from build123d import *

# Parameters (mm, degrees)
ESTRUSIONE_ESTRUSIONE2_DEPTH      = 150
ESTRUSIONE_ESTRUSIONE2_DEPTH_BACK = 150
ESTRUSIONE_ESTRUSIONE3_DEPTH      = 3.3
ESTRUSIONE_ESTRUSIONE3_DEPTH_BACK = 303.3
SCHIZZO3_W                        = 6.5
SCHIZZO3_H                        = 6.5
SCHIZZO11_W                       = 60
SCHIZZO11_H                       = 4
ESTRUSIONE_ESTRUSIONE10_DEPTH     = 2.5
ESTRUSIONE_ESTRUSIONE11_DEPTH     = 2.5
SCHIZZO11_8_W                     = 43
SCHIZZO11_8_H                     = 1.75
ESTRUSIONE_ESTRUSIONE12_DEPTH     = 4.5
SCHIZZO13_W                       = 213
SCHIZZO13_H                       = 5
ESTRUSIONE_ESTRUSIONE13_DEPTH     = 300
SCHIZZO15_W                       = 7
SCHIZZO15_H                       = 5
ESTRUSIONE_ESTRUSIONE14_DEPTH     = 4
SCHIZZO16_W                       = 213
SCHIZZO16_H                       = 5
ESTRUSIONE_ESTRUSIONE15_DEPTH     = 300
RIPETIZIONE_A_L2_COUNT            = 2
RIPETIZIONE_A_L2_PITCH            = 304
SPECCHIA2_COPY_1_SKETCH_W         = 7
SPECCHIA2_COPY_1_SKETCH_H         = 5
SPECCHIA2_COPY_1_DEPTH            = 4
SPECCHIA2_COPY_2_SKETCH_W         = 213
SPECCHIA2_COPY_2_SKETCH_H         = 5
SPECCHIA2_COPY_2_DEPTH            = 300
SCHIZZO17_W                       = 83.15
SCHIZZO17_H                       = 226.3
TAGLIO_ESTRUSIONE1_DEPTH          = 404
SCHIZZO18_W                       = 226.3
SCHIZZO18_H                       = 7
SCHIZZO18_H_2                     = 282
TAGLIO_ESTRUSIONE2_DEPTH          = 404
SCHIZZO23_W                       = 221.3
SCHIZZO23_H                       = 4
SCHIZZO23_H_2                     = 1.75
TAGLIO_ESTRUSIONE7_DEPTH          = 404
SCHIZZO24_W                       = 20
SCHIZZO24_H                       = 221.3
TAGLIO_ESTRUSIONE8_DEPTH          = 404


with BuildPart() as part:
    # Schizzo2 → Estrusione-Estrusione2 (new, two sides: drawn at the far end of the back side and taken through both)
    with BuildSketch(Plane(origin=(0, 0, 0), x_dir=(1, 0, 0), z_dir=(0, 1, 0)).offset(-ESTRUSIONE_ESTRUSIONE2_DEPTH_BACK)):
        Polygon((-113.15, 106.65), (-113.15, -106.65), (-106.65, -106.65), (-106.65, -113.15), (106.65, -113.15), (106.65, -106.65), (113.15, -106.65), (113.15, 106.65), (106.65, 106.65), (106.65, 113.15), (-106.65, 113.15), (-106.65, 106.65), align=None)
    extrude(amount=ESTRUSIONE_ESTRUSIONE2_DEPTH + ESTRUSIONE_ESTRUSIONE2_DEPTH_BACK)

    # Schizzo3 → Estrusione-Estrusione3 (add, two sides: drawn at the far end of the back side and taken through both)
    with BuildSketch(Plane.XZ.offset(150).offset(-ESTRUSIONE_ESTRUSIONE3_DEPTH_BACK)):
        with Locations((-109.9, 109.9)):
            Rectangle(SCHIZZO3_W, SCHIZZO3_H)
        with Locations((109.9, 109.9)):
            Rectangle(SCHIZZO3_W, SCHIZZO3_H)
        with Locations((109.9, -109.9)):
            Rectangle(SCHIZZO3_W, SCHIZZO3_H)
        with Locations((-109.9, -109.9)):
            Rectangle(SCHIZZO3_W, SCHIZZO3_H)
    extrude(amount=ESTRUSIONE_ESTRUSIONE3_DEPTH + ESTRUSIONE_ESTRUSIONE3_DEPTH_BACK)

    # Schizzo11 → Estrusione-Estrusione10 (add)
    with BuildSketch(Plane(origin=(0, 0, -113.15), x_dir=(-1, 0, 0), z_dir=(0, 0, -1))):
        with Locations((0, 141)):
            Rectangle(SCHIZZO11_W, SCHIZZO11_H)
    estrusione_estrusione10 = extrude(amount=ESTRUSIONE_ESTRUSIONE10_DEPTH)

    # Schizzo11_5 → Estrusione-Estrusione11 (add)
    with BuildSketch(Plane(origin=(0, 0, -113.15), x_dir=(-1, 0, 0), z_dir=(0, 0, -1))):
        Polygon((30, 139), (-30, 139), (-45, 139), (-45, 135.5), (-43, 135.5), (-43, 133.75), (0, 133.75), (43, 133.75), (43, 135.5), (45, 135.5), (45, 139), align=None)
    estrusione_estrusione11 = extrude(amount=ESTRUSIONE_ESTRUSIONE11_DEPTH)

    # Schizzo11_8 → Estrusione-Estrusione12 (add)
    with BuildSketch(Plane(origin=(0, 0, -113.15), x_dir=(-1, 0, 0), z_dir=(0, 0, -1))):
        with Locations((21.5, 132.875)):
            Rectangle(SCHIZZO11_8_W, SCHIZZO11_8_H)
        with Locations((-21.5, 132.875)):
            Rectangle(SCHIZZO11_8_W, SCHIZZO11_8_H)
        Polygon((-43, 135.5), (-45, 135.5), (-45, 132), (-43, 132), (-43, 133.75), align=None)
        Polygon((45, 132), (45, 135.5), (43, 135.5), (43, 133.75), (43, 132), align=None)
    estrusione_estrusione12 = extrude(amount=ESTRUSIONE_ESTRUSIONE12_DEPTH)

    # Schizzo13 → Estrusione-Estrusione13 (add)
    with BuildSketch(Plane(origin=(0, 0, -115.65), x_dir=(-1, 0, 0), z_dir=(0, 0, -1))):
        with Locations((-0.15, 136.25)):
            Rectangle(SCHIZZO13_W, SCHIZZO13_H)
    estrusione_estrusione13 = extrude(amount=ESTRUSIONE_ESTRUSIONE13_DEPTH)

    # Schizzo15 → Estrusione-Estrusione14 (add)
    with BuildSketch(Plane(origin=(0, 0, -415.65), x_dir=(-1, 0, 0), z_dir=(0, 0, -1))):
        with Locations((-98.15, 136.25)):
            Rectangle(SCHIZZO15_W, SCHIZZO15_H)
        with Locations((98.15, 136.25)):
            Rectangle(SCHIZZO15_W, SCHIZZO15_H)
    estrusione_estrusione14 = extrude(amount=ESTRUSIONE_ESTRUSIONE14_DEPTH)

    # Schizzo16 → Estrusione-Estrusione15 (add)
    with BuildSketch(Plane(origin=(0, 0, -419.65), x_dir=(-1, 0, 0), z_dir=(0, 0, -1))):
        with Locations((-0.15, 136.25)):
            Rectangle(SCHIZZO16_W, SCHIZZO16_H)
    estrusione_estrusione15 = extrude(amount=ESTRUSIONE_ESTRUSIONE15_DEPTH)

    # Ripetizione a L2: Estrusione-Estrusione14, Estrusione-Estrusione15 ×2
    with Locations(*[(0, 0, -i * RIPETIZIONE_A_L2_PITCH) for i in range(1, RIPETIZIONE_A_L2_COUNT)]):
        add(estrusione_estrusione14)
        add(estrusione_estrusione15)

    # Specchia2: Estrusione-Estrusione10, Estrusione-Estrusione11, Estrusione-Estrusione12, Estrusione-Estrusione13, Estrusione-Estrusione14, Estrusione-Estrusione15 across plane
    add(estrusione_estrusione10.mirror(Plane.XY))
    add(estrusione_estrusione11.mirror(Plane.XY))
    add(estrusione_estrusione12.mirror(Plane.XY))
    add(estrusione_estrusione13.mirror(Plane.XY))
    add(estrusione_estrusione14.mirror(Plane.XY))
    add(estrusione_estrusione15.mirror(Plane.XY))

    # Specchia2 copy 1 sketch → Specchia2 copy 1 (add)
    with BuildSketch(Plane(origin=(0, 0, 719.65), x_dir=(-1, 0, 0), z_dir=(0, 0, 1))):
        with Locations((-98.15, -136.25)):
            Rectangle(SPECCHIA2_COPY_1_SKETCH_W, SPECCHIA2_COPY_1_SKETCH_H)
        with Locations((98.15, -136.25)):
            Rectangle(SPECCHIA2_COPY_1_SKETCH_W, SPECCHIA2_COPY_1_SKETCH_H)
    extrude(amount=SPECCHIA2_COPY_1_DEPTH)

    # Specchia2 copy 2 sketch → Specchia2 copy 2 (add)
    with BuildSketch(Plane(origin=(0, 0, 723.65), x_dir=(-1, 0, 0), z_dir=(0, 0, 1))):
        with Locations((-0.15, -136.25)):
            Rectangle(SPECCHIA2_COPY_2_SKETCH_W, SPECCHIA2_COPY_2_SKETCH_H)
    extrude(amount=SPECCHIA2_COPY_2_DEPTH)

    # Schizzo17 → Taglio-Estrusione1 (cut)
    with BuildSketch(Plane(origin=(0, 150, 0), x_dir=(1, 0, 0), z_dir=(0, 1, 0))):
        with Locations((-71.575, 0)):
            Rectangle(SCHIZZO17_W, SCHIZZO17_H)
        with Locations((71.575, 0)):
            Rectangle(SCHIZZO17_W, SCHIZZO17_H)
    extrude(amount=-TAGLIO_ESTRUSIONE1_DEPTH, mode=Mode.SUBTRACT)


with BuildPart() as taglio_estrusione1_piece_1:
    # of the separate pieces the step leaves, piece 1, a body of its own (taglio_estrusione1_pieces)
    add(part.part.solids().sort_by_distance((106.65, 138.75, 723.65))[0])

    # Schizzo18 → Taglio-Estrusione2 (cut)
    with BuildSketch(Plane(origin=(30, 0, 0), x_dir=(0, 0, -1), z_dir=(1, 0, 0))):
        with Locations((0, 146.5)):
            Rectangle(SCHIZZO18_W, SCHIZZO18_H)
        with Locations((0, -9)):
            Rectangle(SCHIZZO18_W, SCHIZZO18_H_2)
    extrude(amount=-TAGLIO_ESTRUSIONE2_DEPTH, mode=Mode.SUBTRACT)

    # Schizzo23 → Taglio-Estrusione7 (cut)
    with BuildSketch(Plane(origin=(30, 0, 0), x_dir=(0, 0, -1), z_dir=(1, 0, 0))):
        with Locations((0, 141)):
            Rectangle(SCHIZZO23_W, SCHIZZO23_H)
        with Locations((0, 132.875)):
            Rectangle(SCHIZZO23_W, SCHIZZO23_H_2)
    extrude(amount=-TAGLIO_ESTRUSIONE7_DEPTH, mode=Mode.SUBTRACT)

    # Schizzo24 → Taglio-Estrusione8 (cut)
    with BuildSketch(Plane(origin=(0, 139, 0), x_dir=(1, 0, 0), z_dir=(0, 1, 0))):
        with Locations((-20, 0)):
            Rectangle(SCHIZZO24_W, SCHIZZO24_H)
        with Locations((20, 0)):
            Rectangle(SCHIZZO24_W, SCHIZZO24_H)
    extrude(amount=-TAGLIO_ESTRUSIONE8_DEPTH, mode=Mode.SUBTRACT)


with BuildPart() as taglio_estrusione1_piece_2:
    # of the separate pieces the step leaves, piece 2, a body of its own (taglio_estrusione1_pieces)
    add(part.part.solids().sort_by_distance((-106.65, 150, 113.15))[0])


with BuildPart() as taglio_estrusione1_piece_3:
    # of the separate pieces the step leaves, piece 3, a body of its own (taglio_estrusione1_pieces)
    add(part.part.solids().sort_by_distance((-106.65, 150, -106.65))[0])


with BuildPart() as taglio_estrusione1_piece_4:
    # of the separate pieces the step leaves, piece 4, a body of its own (taglio_estrusione1_pieces)
    add(part.part.solids().sort_by_distance((113.15, 150, -106.65))[0])


with BuildPart() as taglio_estrusione1_piece_5:
    # of the separate pieces the step leaves, piece 5, a body of its own (taglio_estrusione1_pieces)
    add(part.part.solids().sort_by_distance((106.65, 150, 113.15))[0])


solid = taglio_estrusione1_piece_1.part
Build history of the part. All positions in model axes, mm. A direction names the side the tool comes from. Round coordinates to 2 decimals unless told otherwise and drop trailing zeros. Loops run counter-clockwise (first coordinate to the right, second up) from the corner with the lowest first, then second, coordinate; pieces in that order, holes last. Notation, with made-up numbers: (8.5, 27) -> (19.5, 27) arc R25 ccw to (19.5, 45) -> close; hole circle Ø3 at (-17.5, 84.5). An arc over 180 degrees is marked (long way). Answer in a Markdown table with one row per item.
Item 1: Saw through at B-B (x = 72). Write the cut outline in (y, z), and give its area (3 significant figures).
Answers below:
| item | result |
|---|---|
| outline | (133.75, -1023.65) -> (138.75, -1023.65) -> (138.75, -723.65) -> (133.75, -723.65) -> close; (133.75, -719.65) -> (138.75, -719.65) -> (138.75, -419.65) -> (133.75, -419.65) -> close; (133.75, -415.65) -> (138.75, -415.65) -> (138.75, -115.65) -> (133.75, -115.65) -> close; (133.75, 115.65) -> (138.75, 115.65) -> (138.75, 415.65) -> (133.75, 415.65) -> close; (133.75, 419.65) -> (138.75, 419.65) -> (138.75, 719.65) -> (133.75, 719.65) -> close; (133.75, 723.65) -> (138.75, 723.65) -> (138.75, 1023.65) -> (133.75, 1023.65) -> close |
| area | 9,000 mm² |
Item 2: Which spindle directions (+Z, -Z, +X, -X, +Y, -Y) get a long thin tool onto all of the face, cutting with end or side? Do faces 1 (the flat face through (2, 138.75, 563)), 2 (the flat face through (2, 138.75, -563)), 3 (the flat face through (2, 133.75, -563)). Say none if no direction does.
Answers below:
| item | result |
|---|---|
| face 1 | +Z, +X, -X, +Y |
| face 2 | -Z, +X, -X, +Y |
| face 3 | -Z, +X, -X, -Y |
Item 3: Pin check, flat tips, straight feed: pin 1 (12 mm diameter, centred on x = 19.5, z = 669.5, fed in from +Y); pin 2 (1.9 mm diameter, centred on x = 15, y = 133, fed in from +Z); pin 3 (1.2 mm diameter, centred on y = 135.5, z = 721, fed in from +X); pin 4 (12 mm diameter, centred on x = -8, z = 288.5, fed in from -Y). Stop position of each tip, or through.
Answers below:
| item | result |
|---|---|
| pin 1 | stops at y = 138.75 |
| pin 2 | stops at z = 1023.65 |
| pin 3 | stops at x = 101.65 |
| pin 4 | stops at y = 133.75 |
Item 4: Drill centre lines: L1, parallel to Z at x = -43, y = 134; L2, parallel to Z at x = -88, y = 138.25; L3, parallel to Z at x = -3, y = 135.5. Where is each one in solid material? Low to high. Write a range as [from, to].
Answers below:
| item | result |
|---|---|
| L1 | z = [-1023.65, -723.65], [-719.65, -419.65], [-415.65, -113.15], [113.15, 415.65], [419.65, 719.65], [723.65, 1023.65] |
| L2 | z = [-1023.65, -723.65], [-719.65, -419.65], [-415.65, -115.65], [115.65, 415.65], [419.65, 719.65], [723.65, 1023.65] |
| L3 | z = [-1023.65, -723.65], [-719.65, -419.65], [-415.65, 415.65], [419.65, 719.65], [723.65, 1023.65] |
Item 5: Saw through at C-C (z = 314.5). Write the cut outline in (x, y).
Answers below:
| item | result |
|---|---|
| outline | (-106.35, 133.75) -> (106.65, 133.75) -> (106.65, 138.75) -> (-106.35, 138.75) -> close |
Item 6: Saw through at D-D (z = 52.5). Write the cut outline in (x, y).
Answers below:
| item | result |
|---|---|
| outline | (-10, 133.75) -> (10, 133.75) -> (10, 139) -> (-10, 139) -> close |
Item 7: Saw through at A-A (y = 141). Write the cut outline in (x, z).
Answers below:
| item | result |
|---|---|
| outline | (-30, -115.65) -> (30, -115.65) -> (30, -110.65) -> (-30, -110.65) -> close; (-30, 110.65) -> (30, 110.65) -> (30, 115.65) -> (-30, 115.65) -> close |
